Geometry check sheet. Reference: the model listing, model coordinates, mm. Face numbers are marked on the shaded views. Give positions to 0.01 mm unless a question says otherwise; leave off trailing zeros. Order: outer loops, then holes, each group sorted by start corner. A loop starts at its lowest first (then second) coordinate and runs counter-clockwise, first axis right, second up. Notation, with made-up numbers: M -11,55.25 L 24,55.25 A17 ccw 24,80.25 Z; hole C -1,-25 d1. An arc over 180 degrees is marked long. Put each result on its own line as item: value. Start each with the question number.
Q1. Section check C-C on z = 81. Record the cut outline in (x, y).
Q2. Section check B-B on y = -27. Record the cut outline in (x, z).
Q3. Section check D-D on x = 78.5. Record the cut outline in (y, z), then the cut area to 3 significant figures.
Q4. Material ranges on L1, parallel to Y at x = -11, z = 64.5; L2, parallel to Z at x = 80, y = -5.5; L3, parallel to X at y = -1.5, z = 136, recorded low to high.
Q5. Go/stop test with flat-tipped pins: pin 1 (10 mm diameter, centred on x = -1.5, z = 167.5, fed in from -Y); pin 2 (1 mm diameter, centred on x = 65.5, z = 147.5, fed in from -Y); pin 3 (2.5 mm diameter, centred on y = -1.5, z = 140, fed in from -X). Record where each tip stops, or that it passes through.
Q6. Mould release check, pull along Y, two halves, no side actions. Record for the marked faces 1 and 2: +Y half, -Y half, draft (parallel to the pull), parting line (faces both ways), or undercut.
Q7. Section check A-A on x = -28. Record the cut outline in (y, z).
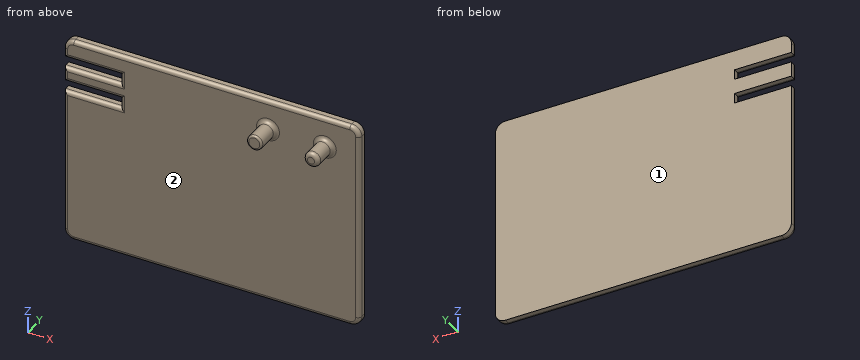
```python
from build123d import *

# Parameters (mm, degrees)
F1_DEPTH = 9
F2_R     = 7.5
F3_DEPTH = 25
F4_W     = 57
F4_H     = 10
F5_DEPTH = 25
F6_R     = 2
F7_R     = 4
F8_R     = 4


with BuildPart() as f1:
    # F0 (on Front) → F1 (new body)
    with BuildSketch(Plane.XZ):
        with BuildLine():
            Line((231.2582800984, 190.805722177), (-45.7417199016, 190.805722177))
            ThreePointArc((-45.7417199016, 190.805722177), (-52.8127877134, 187.8767899889), (-55.7417199016, 180.805722177))
            Line((-55.7417199016, 180.805722177), (-55.7417199016, -9.194277823))
            ThreePointArc((-55.7417199016, -9.194277823), (-52.8127877134, -16.2653456348), (-45.7417199016, -19.194277823))
            Line((-45.7417199016, -19.194277823), (231.2582800984, -19.194277823))
            ThreePointArc((231.2582800984, -19.194277823), (238.3293479103, -16.2653456348), (241.2582800984, -9.194277823))
            Line((241.2582800984, -9.194277823), (241.2582800984, 180.805722177))
            ThreePointArc((241.2582800984, 180.805722177), (238.3293479103, 187.8767899889), (231.2582800984, 190.805722177))
        make_face()
    extrude(amount=F1_DEPTH)

    # F2 (on face) → F3 (join)
    with BuildSketch(Plane.XZ.offset(9)):
        with Locations((149.2582800984, 160.805722177)):
            Circle(F2_R)
        with Locations((206.2582800984, 160.805722177)):
            Circle(F2_R)
    extrude(amount=F3_DEPTH)

    # F4 (on face) → F5 (cut)
    with BuildSketch(Plane.XZ.offset(9)):
        with Locations((-27.2417199016, 165.805722177)):
            Rectangle(F4_W, F4_H)
        with Locations((-27.2417199016, 140.805722177)):
            Rectangle(F4_W, F4_H)
    extrude(amount=-F5_DEPTH, mode=Mode.SUBTRACT)

    # F6
    f6_edges = [f1.edges().sort_by_distance(p)[0] for p in [
        (141.75828, -34, 160.805722),
    ]]
    fillet(f6_edges, radius=F6_R)

    # F7
    f7_edges = [f1.edges().sort_by_distance(p)[0] for p in [
        (198.75828, -34, 160.805722),
    ]]
    fillet(f7_edges, radius=F7_R)

    # F8
    f8_edges = [f1.edges().sort_by_distance(p)[0] for p in [
        (143.75828, -34, 160.805722),
        (141.75828, -32, 160.805722),
        (238.329348, -9, 187.87679),
        (241.25828, -9, 85.805722),
        (238.329348, -9, -16.265346),
        (92.75828, -9, -19.194278),
        (-52.812788, -9, -16.265346),
        (-55.74172, -9, 63.305722),
        (-27.24172, -9, 135.805722),
        (1.25828, -9, 140.805722),
        (-27.24172, -9, 145.805722),
        (-55.74172, -9, 153.305722),
        (-27.24172, -9, 160.805722),
        (1.25828, -9, 165.805722),
        (-27.24172, -9, 170.805722),
        (-55.74172, -9, 175.805722),
        (-52.812788, -9, 187.87679),
        (92.75828, -9, 190.805722),
        (141.75828, -9, 160.805722),
        (198.75828, -9, 160.805722),
    ]]
    fillet(f8_edges, radius=F8_R)


solid = f1.part
```
Results found:
1. outline: M -55.74,-5 A4 ccw -51.74,-9 L 237.26,-9 A4 ccw 241.26,-5 L 241.26,0 L -55.74,0 Z
2. outline: C 149.26,160.81 d15; C 206.26,160.81 d15
3. outline: M -9,-15.19 A4 ccw -5,-19.19 L 0,-19.19 L 0,190.81 L -5,190.81 A4 ccw -9,186.81 Z
3. area: 1,880 mm^2
4. L1: y = -9 to 0
4. L2: z = -19.16 to 190.77
4. L3: x = 1.26 to 241.26
5. pin 1: stops at y = -8.59
5. pin 2: stops at y = -9
5. pin 3: stops at x = 1.26
6. face 1: +Y half
6. face 2: -Y half
7. outline: M -9,-15.19 A4 ccw -5,-19.19 L 0,-19.19 L 0,135.81 L -5,135.81 A4 ccw -9,131.81 Z; M -9,149.81 A4 ccw -5,145.81 L 0,145.81 L 0,160.81 L -5,160.81 A4 ccw -9,156.81 Z; M -9,174.81 A4 ccw -5,170.81 L 0,170.81 L 0,190.81 L -5,190.81 A4 ccw -9,186.81 Z
